The listing builds one solid part. Answer for the finished solid, in the listing's coordinates (mm). Round coordinates to 2 decimals unless told otherwise and drop trailing zeros. Write each loop counter-clockwise with the first axis right and the second up, starting at its lowest first coordinate (ties: lowest second). Pieces come first, ordered by that corner, then holes.
Item 1: Each of these flat-tipped pins is pushed along its axis until it touches: pin 1 (2 mm diameter, centred on x = 23, z = 6, fed in from +Y); pin 2 (3 mm diameter, centred on y = 76.5, z = 8.5, fed in from +X); pin 3 (6 mm diameter, centred on x = 35, y = 2, fed in from -Z). Where does it stop, or does it pass through?
Item 2: Find section B-B on y = 30. Give the vertices of the cut face in (x, z).
Item 3: Find the intervals of material crossed by probe 1 along Y at (x, z) = (15, 3.75); probe 2 along Y at (x, z) = (37, 5.5); probe 3 along X at (y, z) = (113.5, 3.25), in increasing order.
Item 4: Find section C-C on x = 0. Give the vertices of the cut face in (y, z).
```python
from build123d import *

# Parameters (mm, degrees)
EXTRUDE_1_DEPTH = 10


with BuildPart() as part:
    # 草图1 → 凸台-拉伸1 (new body)
    with BuildSketch(Plane.XY):
        with BuildLine():
            Line((26.783972095, 133.739971334), (26.847812167, 133.883151585))
            ThreePointArc((26.847812167, 133.883151585), (66.392800103, 149.097978029), (81.71089656, 109.59287791))
            Line((81.71089656, 109.59287791), (83.99950279, 108.586755885))
            ThreePointArc((83.99950279, 108.586755885), (67.327208125, 151.41822318), (24.49574083, 134.745928515))
            Line((24.49574083, 134.745928515), (26.783972095, 133.739971334))
        make_face()
        with BuildLine():
            ThreePointArc((-27.46327475, 12.073464291), (-27.431635829, 12.145178293), (-27.399809643, 12.216809384))
            Line((-27.399809643, 12.216809384), (26.783972095, 133.739971334))
            Line((26.783972095, 133.739971334), (24.49574083, 134.745928515))
            Line((24.49574083, 134.745928515), (-29.75188098, 13.079586315))
            Line((-29.75188098, 13.079586315), (-27.46327475, 12.073464291))
        make_face()
        with BuildLine():
            Line((81.647431453, 109.449532816), (27.463649715, -12.073629134))
            Line((27.463649715, -12.073629134), (29.75188098, -13.079586315))
            Line((29.75188098, -13.079586315), (83.99950279, 108.586755885))
            Line((83.99950279, 108.586755885), (81.71089656, 109.59287791))
            ThreePointArc((81.71089656, 109.59287791), (81.679257639, 109.521163908), (81.647431453, 109.449532816))
        make_face()
        with BuildLine():
            Line((27.463649715, -12.073629134), (27.399809643, -12.216809384))
            ThreePointArc((27.399809643, -12.216809384), (-12.145178293, -27.431635829), (-27.46327475, 12.073464291))
            Line((-27.46327475, 12.073464291), (-29.75188098, 13.079586315))
            ThreePointArc((-29.75188098, 13.079586315), (-13.079586315, -29.75188098), (29.75188098, -13.079586315))
            Line((29.75188098, -13.079586315), (27.463649715, -12.073629134))
        make_face()
    extrude(amount=EXTRUDE_1_DEPTH)


solid = part.part
```
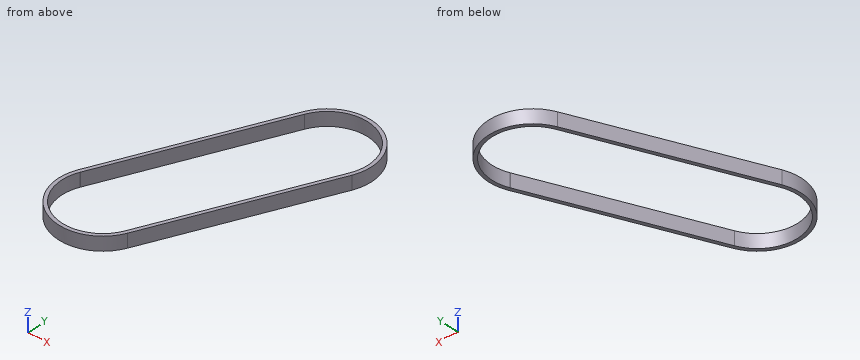
Check values:
1. pin 1: stops at y = 133.63
1. pin 2: stops at x = 70.36
1. pin 3: stops at z = 0
2. outline: (-22.21, 0) - (-19.47, 0) - (-19.47, 10) - (-22.21, 10) - close; (46.22, 0) - (48.96, 0) - (48.96, 10) - (46.22, 10) - close
3. probe 1: y = -28.83 to -25.98, 107.31 to 113.45
3. probe 2: y = 3.18 to 9.31, 146.21 to 149.21
3. probe 3: x = 15.02 to 17.76, 83.11 to 85.7
4. outline: (-32.5, 0) - (-30, 0) - (-30, 10) - (-32.5, 10) - close; (73.67, 0) - (79.81, 0) - (79.81, 10) - (73.67, 10) - close
